from build123d import *

# Parameters (mm, degrees)
SKETCH002_W = 348
SKETCH002_H = 204
SKETCH001_W = 352.462198
SKETCH001_H = 208.462198
THICKNESS_T = -3
FILLET_R    = 2.7


with BuildPart() as part:
    # Sketch002 → AdditiveLoft section 0
    with BuildSketch(Plane.XY.offset(52)):
        Rectangle(SKETCH002_W, SKETCH002_H)
    # Sketch001 → AdditiveLoft section 1
    with BuildSketch(Plane.XY.offset(31)):
        Rectangle(SKETCH001_W, SKETCH001_H)
    loft()

    # Thickness
    thickness_openings = [part.faces().sort_by_distance(p)[0] for p in [
        (0, 0, 31),
    ]]
    offset(amount=THICKNESS_T, openings=thickness_openings, kind=Kind.INTERSECTION)

    # Fillet
    fillet_edges = [part.edges().sort_by_distance(p)[0] for p in [
        (-175.115549, -103.115549, 41.5),
        (0, -102, 52),
        (-174, 0, 52),
        (0, 102, 52),
        (175.115549, -103.115549, 41.5),
        (174, 0, 52),
        (175.115549, 103.115549, 41.5),
        (-175.115549, 103.115549, 41.5),
    ]]
    fillet(fillet_edges, radius=FILLET_R)


solid = part.part
Model file for the job. Use its own axes, mm. A direction names the side the tool comes from. Give positions to 0.01 mm unless a question says otherwise; leave off trailing zeros. Answer as CSV lines item,"result".
1. Pin check, flat tips, straight feed: pin 1 (4 mm diameter, centred on y = 4, z = 41, fed in from +X); pin 2 (5 mm diameter, centred on y = -49.5, z = 48, fed in from -X); pin 3 (4 mm diameter, centred on x = -40, z = 46, fed in from +Y). Stop position of each tip, or through.
Responses:
pin 1,"stops at x = 175.38"
pin 2,"stops at x = -174.69"
pin 3,"stops at y = 102.85"
2. Drill centre lines: L1, parallel to Z at x = -18, y = 43; L2, parallel to Y at x = 107, z = 48; L3, parallel to X at y = -20.5, z = 46.5. Where is each one in solid material? Low to high. Write a range as [from, to].
Responses:
L1,"z = [49, 52]"
L2,"y = [-102.42, -99.41], [99.41, 102.42]"
L3,"x = [-174.58, -171.57], [171.57, 174.58]"
3. Two-plate mould, pull along Y, no slides. Class faces 1 (the face through (-2.42, -100.27, 39.87)), 2 (the face through (-4, 1, 52)): +Y half, -Y half, draft (parallel to the pull), parting line (faces both ways), or undercut.
Responses:
face 1,"undercut"
face 2,"draft"
4. 3-axis set-ups, long thin cutter, end or side, ignore diameter. For faces 3 (the face through (172.27, -1.42, 39.87)), 4 (the face through (43, 103, 31)): which of +Z, -Z, +X, -X, +Y, -Y reach the whole face in a straight line?
Responses:
face 3,"-Z"
face 4,"-Z, +X, -X, +Y, -Y"
